For this review, use the dimensioned drawing (mm, ordinates from the lowest corner) and the shaded views. Coordinates: 2 decimals unless noted, no trailing zeros. Loops run counter-clockwise (first coordinate to the right, second up) from the corner with the lowest first, then second, coordinate; pieces in that order, holes last. Notation, with made-up numbers: M -27,-9.5 L -10,-9.5 A21 cw -10,1.5 Z; hole C 34,61 d10. An arc over 180 degrees is marked long. Use CSV: the item, a comma, the result in double quotes. Start each with the question number.
1. Add section B-B, the plane z = 7.75. Write out the cut boundary in (x, y) (3 decimals), then the cut area to 3 significant figures.
2. For L1, parallel to X at y = 8.5, z = 8.5; L2, parallel to X at y = 10.25, z = 7; L3, parallel to Y at x = 527.05, z = 3.5, list the stretches that pass through material, from the lowest coordinate up.
3. Clearance check with a flat-ended pin moving along its axis: P1, Ø6.5, axis at x = 276.225, y = 9.525, coming from the +Z side. State where the tip first meets the part, or that it passes through.
4. Add section A-A, the plane x = 527.05. Write out the cut boundary in (y, z), then the cut area to 4 significant figures.
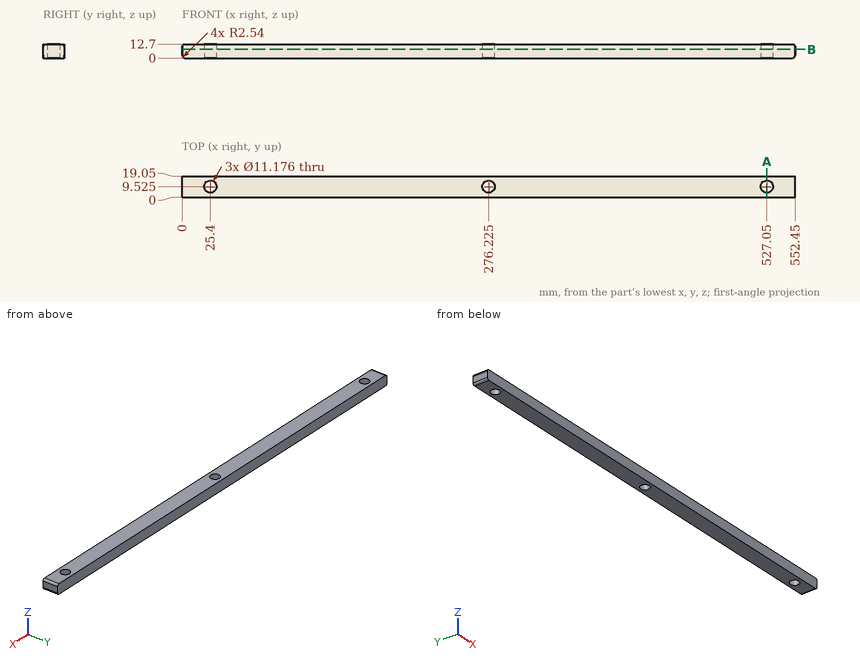
Computed:
1,outline,"M 0,0 L 552.45,0 L 552.45,19.05 L 0,19.05 Z; hole C 25.4,9.525 d11.176; hole C 276.225,9.525 d11.176; hole C 527.05,9.525 d11.176"
1,area,"10,200 mm^2"
2,L1,"x = 0 to 19.91, 30.89 to 270.73, 281.72 to 521.56, 532.54 to 552.45"
2,L2,"x = 0 to 19.86, 30.94 to 270.68, 281.77 to 521.51, 532.59 to 552.45"
2,L3,"y = 0 to 3.94, 15.11 to 19.05"
3,P1,"passes through"
4,outline,"M 0,0 L 3.94,0 L 3.94,12.7 L 0,12.7 Z; M 15.11,0 L 19.05,0 L 19.05,12.7 L 15.11,12.7 Z"
4,area,"100.0 mm^2"
